```python
from build123d import *

# Parameters (mm, degrees)
F1_DEPTH = 4.1402
F3_D     = 5.1054
F4_SIZE  = 0.254


with BuildPart() as f1:
    # F0 (on Front) → F1 (new body)
    with BuildSketch(Plane.XZ):
        Polygon((-3.1175517919, 5.6158314171), (-6.4222285665, 0.1080366591), (-3.3046767746, -5.5077947579), (3.1175517919, -5.6158314171), (6.4222285665, -0.1080366591), (3.3046767746, 5.5077947579), align=None)
    extrude(amount=F1_DEPTH)

    # F3 (through all)
    with Locations(Plane.XZ.offset(4.1402)):
        with Locations((0, 0)):
            Hole(F3_D / 2)

    # F4
    f4_edges = [f1.edges().sort_by_distance(p)[0] for p in [
        (-4.76989, -4.1402, 2.861934),
        (0.093562, -4.1402, 5.561813),
        (4.863453, -4.1402, 2.699879),
        (4.76989, -4.1402, -2.861934),
        (-0.093562, -4.1402, -5.561813),
        (-4.863453, -4.1402, -2.699879),
        (-4.863453, 0, -2.699879),
        (-4.76989, 0, 2.861934),
        (0.093562, 0, 5.561813),
        (4.863453, 0, 2.699879),
        (4.76989, 0, -2.861934),
        (-0.093562, 0, -5.561813),
    ]]
    chamfer(f4_edges, length=F4_SIZE)


solid = f1.part
```
Geometry: final body of the model. Coordinates: model frame, mm. Round coordinates to 2 decimals unless told otherwise and drop trailing zeros. Write each loop counter-clockwise with the first axis right and the second up, starting at its lowest first coordinate (ties: lowest second). Pieces come first, ordered by that corner, then holes. Notation, with made-up numbers: (23, 78) -> (35, 78) arc R21 ccw to (35, 90) -> close; hole circle Ø4 at (-22, 26). An arc over 180 degrees is marked (long way). Use CSV: the item, a comma, the result in double quotes. Start each with the question number.
Q1. Line query: L1, parallel to Z at x = -0.5, y = -3.05; L2, parallel to X at y = -0.85, z = -0.5; L3, parallel to Z at x = 1.75, y = -1.55. Output: solid intervals per line, ascending.
Q2. Section B-B (x = 0). Return loops of the section in (y, z).
Q3. Section A-A (y = -3.1). Return loops of the section in (x, z), plus the area to 3 significant figures.
Q4. Section C-C (z = 1.25). Return loops of the section in (x, y).
Q5. Section D-D (x = -3.75). Return loops of the section in (y, z).
Q6. Pull-direction query (Z, two-part tool) for faces 1 (the face through (-2.435, -2.041, 0.767)), 2 (the face through (3, -4.14, 0)), 3 (the face through (4.747, -2.045, -2.9)); classes: pulls with the +Z half, pulls with the -Z half, needs draft (parallel to the pull), parting line crosses it, or undercut.
Q7. First-contact query: pin 1 Ø1 at (y, z) = (-3.5, -3) entering from +X; pin 2 Ø1 at (x, y) = (3, -1) entering from +Z; pin 3 Ø1.5 at (x, y) = (-4.5, -3) entering from +Z. Flat tips, straight axial feed; report the tip coordinate or a pass-through.
Result sheet:
1,L1,"-5.55 to -2.5, 2.5 to 5.57"
1,L2,"-6.08 to -2.5, 2.5 to 6.19"
1,L3,"-5.59 to -1.86, 1.86 to 5.53"
2,outline,"(-4.14, -5.31) -> (-3.89, -5.56) -> (-0.25, -5.56) -> (0, -5.31) -> (0, -2.55) -> (-4.14, -2.55) -> close; (-4.14, 2.55) -> (0, 2.55) -> (0, 5.31) -> (-0.25, 5.56) -> (-3.89, 5.56) -> (-4.14, 5.31) -> close"
3,outline,"(-6.42, 0.11) -> (-3.3, -5.51) -> (3.12, -5.62) -> (6.42, -0.11) -> (3.3, 5.51) -> (-3.12, 5.62) -> close; hole circle Ø5.11 at (0, 0)"
3,area,"86.7 mm²"
4,outline,"(-5.74, -3.89) -> (-5.44, -4.14) -> (-2.23, -4.14) -> (-2.23, 0) -> (-5.44, 0) -> (-5.74, -0.25) -> close; (2.23, -4.14) -> (5.38, -4.14) -> (5.67, -3.89) -> (5.67, -0.25) -> (5.38, 0) -> (2.23, 0) -> close"
5,outline,"(-4.14, -4.18) -> (-3.89, -4.71) -> (-0.25, -4.71) -> (0, -4.18) -> (0, 4.07) -> (-0.25, 4.56) -> (-3.89, 4.56) -> (-4.14, 4.07) -> close"
6,face 1,"undercut"
6,face 2,"needs draft"
6,face 3,"pulls with the -Z half"
7,pin 1,"x = 4.99"
7,pin 2,"z = 5.52"
7,pin 3,"z = 4.56"
